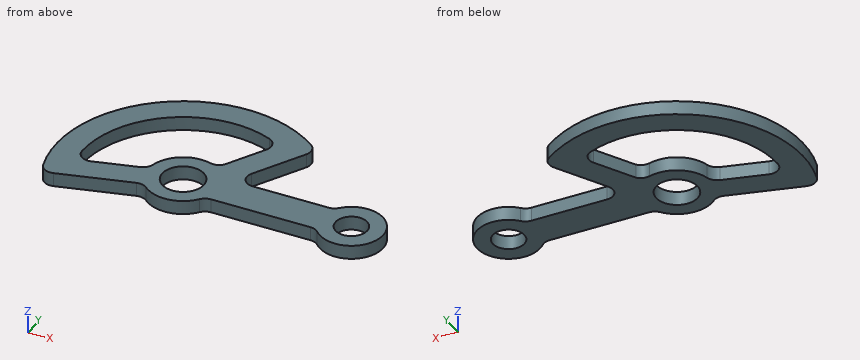
from build123d import *

# Parameters (mm, degrees)
SKETCH2_R           = 8
SKETCH2_R_2         = 10.5
BOSS_EXTRUDE2_DEPTH = 7


with BuildPart() as part:
    # Sketch2 → Boss-Extrude2 (new body)
    with BuildSketch(Plane.XY):
        with BuildLine():
            ThreePointArc((18.734993995, -9), (16.136917784, -9.591673087), (14.051245496, -11.25))
            ThreePointArc((14.051245496, -11.25), (1.588158791, -17.929800658), (-11.855019266, -13.544685977))
            ThreePointArc((-11.855019266, -13.544685977), (-14.447084602, -12.215655673), (-17.359606625, -12.264026344))
            Line((-17.359606625, -12.264026344), (-54.105315802, -22.110009444))
            ThreePointArc((-54.105315802, -22.110009444), (-58.597408553, -21.545250779), (-61.415978011, -18.002156674))
            ThreePointArc((-61.415978011, -18.002156674), (-36.436152523, 52.615651562), (38.455388874, 51.158411493))
            ThreePointArc((38.455388874, 51.158411493), (40.729032534, 47.562011618), (40.04634859, 43.362310416))
            Line((40.04634859, 43.362310416), (25.403411844, 18))
            ThreePointArc((25.403411844, 18), (25.403411844, 12), (30.599564267, 9))
            Line((30.599564267, 9), (68.906523061, 9))
            ThreePointArc((68.906523061, 9), (71.299695166, 9.497934272), (73.295653135, 10.909090909))
            ThreePointArc((73.295653135, 10.909090909), (101, 0), (73.295653135, -10.909090909))
            ThreePointArc((73.295653135, -10.909090909), (71.299695166, -9.497934272), (68.906523061, -9))
            Line((68.906523061, -9), (18.734993995, -9))
        make_face()
        with Locations((85, 0)):
            Circle(SKETCH2_R, mode=Mode.SUBTRACT)
        Circle(SKETCH2_R_2, mode=Mode.SUBTRACT)
        with BuildLine():
            ThreePointArc((10.98874406, 19.033063022), (8.199770085, 17.312416637), (4.922729046, 17.313773094))
            ThreePointArc((4.922729046, 17.313773094), (-9.01320029, 15.580828622), (-17.462949753, 4.364101961))
            ThreePointArc((-17.462949753, 4.364101961), (-19.005575236, 1.612182259), (-21.731018733, 0.023247657))
            Line((-21.731018733, 0.023247657), (-43.447085729, -5.795554958))
            ThreePointArc((-43.447085729, -5.795554958), (-48.652568574, -4.760120042), (-51, 0))
            ThreePointArc((-51, 0), (-28.394096654, 42.364788152), (19.383344125, 47.172936845))
            ThreePointArc((19.383344125, 47.172936845), (22.781794932, 43.559859246), (22.299103121, 38.623179569))
            Line((22.299103121, 38.623179569), (10.98874406, 19.033063022))
        make_face(mode=Mode.SUBTRACT)
    extrude(amount=BOSS_EXTRUDE2_DEPTH)


solid = part.part
Could you check a few things on this model? Use its own coordinates, in mm. Coordinates: 2 decimals unless noted, no trailing zeros. Order: outer loops, then holes, each group sorted by start corner. A loop starts at its lowest first (then second) coordinate and runs counter-clockwise, first axis right, second up. Notation, with made-up numbers: (31, -14) -> (87, -14) arc R21 cw to (87, -4) -> close; hole circle Ø3 at (-33, -28). An arc over 180 degrees is marked (long way). One line per item, written item: value. Start each with the question number.
1) Imagine slicing it at A-A on x = 0. List the corners of the cut face in (y, z) for me.
2) Imagine slicing it at D-D on z = 3.5. List the corners of the cut face in (x, y) for me (3 decimals), plus the area to 3 significant figures.
3) Imagine slicing it at C-C on y = 45.5. List the corners of the cut face in (x, z) for me.
4) If I drill on L1, parallel to Y at x = 0, z = 4; L2, parallel to Y at x = 85, z = 4; L3, parallel to X at y = 11, z = 1.75, over which ranges is the centre line in solid material (lowest first)? Write a range as [from, to].
5) Imagine slicing it at B-B on x = 85. List the corners of the cut face in (y, z) for me, plus the area to 3 significant figures.
6) I'm going to push flat-ended pins straight in: pin 1 (2 mm diameter, centred on x = 49.5, z = 3.5, fed in from +Y); pin 2 (3.5 mm diameter, centred on x = 40, z = 3.5, fed in from -Y); pin 3 (4 mm diameter, centred on x = -4, z = 3, fed in from +Y); pin 4 (17 mm diameter, centred on x = 0, y = 0, fed in from -Z). Where does each tip first touch, or does it pass through?
Answer list:
1. outline: (-18, 0) -> (-10.5, 0) -> (-10.5, 7) -> (-18, 7) -> close; (10.5, 0) -> (18, 0) -> (18, 7) -> (10.5, 7) -> close; (51, 0) -> (64, 0) -> (64, 7) -> (51, 7) -> close
2. outline: (-61.416, -18.002) arc R6 ccw to (-54.105, -22.11) -> (-17.36, -12.264) arc R6 cw to (-11.855, -13.545) arc R18 ccw to (14.051, -11.25) arc R6 cw to (18.735, -9) -> (68.907, -9) arc R6 cw to (73.296, -10.909) arc R16 ccw (long way) to (73.296, 10.909) arc R6 cw to (68.907, 9) -> (30.6, 9) arc R6 cw to (25.403, 18) -> (40.046, 43.362) arc R6 ccw to (38.455, 51.158) arc R64 ccw to start; hole (-51, 0) arc R6 ccw to (-43.447, -5.796) -> (-21.731, 0.023) arc R6 ccw to (-17.463, 4.364) arc R18 cw to (4.923, 17.314) arc R6 ccw to (10.989, 19.033) -> (22.299, 38.623) arc R6 ccw to (19.383, 47.173) arc R51 ccw to start; hole circle Ø21 at (0, 0); hole circle Ø16 at (85, 0)
2. area: 5,160 mm2
3. outline: (-45.01, 0) -> (-23.04, 0) -> (-23.04, 7) -> (-45.01, 7) -> close; (21.68, 0) -> (40.79, 0) -> (40.79, 7) -> (21.68, 7) -> close
4. L1: y = [-18, -10.5], [10.5, 18], [51, 64]
4. L2: y = [-16, -8], [8, 16]
4. L3: x = [-63.05, -49.8], [-14.25, 26.13], [73.38, 96.62]
5. outline: (-16, 0) -> (-8, 0) -> (-8, 7) -> (-16, 7) -> close; (8, 0) -> (16, 0) -> (16, 7) -> (8, 7) -> close
5. area: 112 mm2
6. pin 1: stops at y = 9
6. pin 2: stops at y = -9
6. pin 3: stops at y = 63.97
6. pin 4: passes through
